Build history of the part. All positions in model axes, mm. Face numbers are marked on the shaded views. A direction names the side the tool comes from. Give positions to 0.01 mm unless a question says otherwise; leave off trailing zeros. Order: outer loops, then holes, each group sorted by start corner. A loop starts at its lowest first (then second) coordinate and runs counter-clockwise, first axis right, second up. Notation, with made-up numbers: (-24, 83) - (17, 83) arc R31 cw to (17, 116) - close; hole circle Ø5 at (8, -2). An arc over 180 degrees is marked (long way). Use a Markdown table: item, result. Add a question column.
(1) Flat gauge pins, fed straight in: pin 1 (12 mm diameter, centred on x = 52.5, y = -16, fed in from +Z); pin 2 (1.5 mm diameter, centred on x = 43.5, z = 25, fed in from -Y); pin 3 (6 mm diameter, centred on x = 49.5, z = 27.5, fed in from +Y); pin 4 (2 mm diameter, centred on y = -21.5, z = 8.5, fed in from -X). Where does each tip first touch, or does it go through?
(2) Wall check: line 1 (Y direction, x = 41.5, z = 26); line 2 (X direction, y = -17, z = 28); line 3 (Z direction, x = 56, y = -13). Give the ranges that are in metal, low to high.
(3) Slice it at B-B (x = 34). Write the cut outline in (y, z).
(4) Which spindle directions (+Z, -Z, +X, -X, +Y, -Y) get a long thin tool onto all of the face, cutting with end or side? Do the marked faces 1, 2 and 3. Say none if no direction does.
(5) Slice it at A-A (z = 13). Write the cut outline in (x, y).
(6) Slice it at D-D (y = -30). Write the cut outline in (x, z), then the cut area to 3 significant figures.
(7) Slice it at C-C (y = -20.5). Write the cut outline in (x, z), then the cut area to 3 significant figures.
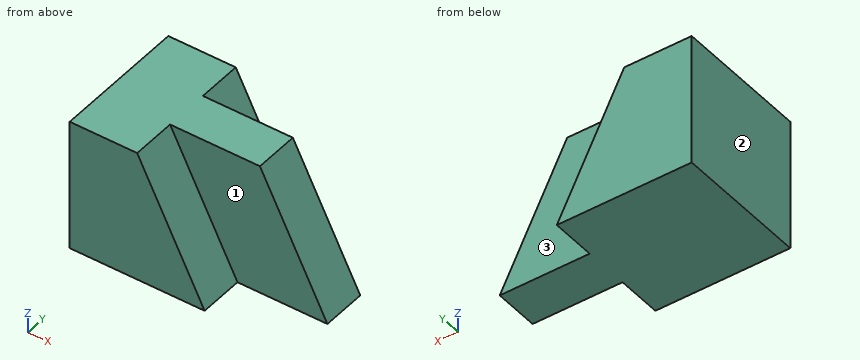
from build123d import *

# Parameters (mm, degrees)
F1_DEPTH = 38.1
F3_DEPTH = 12.7
F5_DEPTH = 12.7


with BuildPart() as f1:
    # F0 (on Front) → F1 (new body)
    with BuildSketch(Plane.XZ):
        Polygon((0, 37.344047), (0, 0), (63.5, 0), (44.45, 37.344047), align=None)
    extrude(amount=F1_DEPTH)

    # F2 (on face) → F3 (cut)
    with BuildSketch(Plane.XZ.offset(38.1)):
        Polygon((44.45, 37.344047), (19.05, 37.344047), (38.1, 0), (63.5, 0), align=None)
    extrude(amount=-F3_DEPTH, mode=Mode.SUBTRACT)

    # F4 (on face) → F5 (cut)
    with BuildSketch(Plane(origin=(0, 0, 0), x_dir=(-1, 0, 0), z_dir=(0, 1, 0))):
        Polygon((-38.1, 0), (-19.05, 37.344047), (-44.45, 37.344047), (-63.5, 0), align=None)
    extrude(amount=-F5_DEPTH, mode=Mode.SUBTRACT)


solid = f1.part
Solution:
| question | item | result |
|---|---|---|
| 1 | pin 1 | z = 33.33 |
| 1 | pin 2 | y = -25.4 |
| 1 | pin 3 | y = -12.7 |
| 1 | pin 4 | x = 0 |
| 2 | line 1 | -25.4 to -12.7 |
| 2 | line 2 | 0 to 49.22 |
| 2 | line 3 | 0 to 14.7 |
| 3 | outline | (-38.1, 0) - (0, 0) - (0, 8.04) - (-12.7, 8.04) - (-12.7, 37.34) - (-25.4, 37.34) - (-25.4, 8.04) - (-38.1, 8.04) - close |
| 4 | face 1 | +Z, +X, -Y |
| 4 | face 2 | +Z, -Z, -X, +Y, -Y |
| 4 | face 3 | +Z, +X, +Y |
| 5 | outline | (0, -38.1) - (31.47, -38.1) - (31.47, -25.4) - (56.87, -25.4) - (56.87, -12.7) - (31.47, -12.7) - (31.47, 0) - (0, 0) - close |
| 6 | outline | (0, 0) - (38.1, 0) - (19.05, 37.34) - (0, 37.34) - close |
| 6 | area | 1,070 mm2 |
| 7 | outline | (0, 0) - (63.5, 0) - (44.45, 37.34) - (0, 37.34) - close |
| 7 | area | 2,020 mm2 |
